```python
from build123d import *

# Parameters (mm, degrees)
F0_W     = 88.9
F0_H     = 57.15
F0_R     = 4.7625
F0_W_2   = 85.160196
F0_H_2   = 10.460668
F1_DEPTH = 3.175
F0_W_3   = 95.25
F0_H_3   = 63.5
F2_DEPTH = 19.05


with BuildPart() as f1:
    # F0 (on Top) → F1 (new body)
    with BuildSketch(Plane.XY):
        Rectangle(F0_W, F0_H)
        Polygon((-25.4, 3.175), (-25.4, 11.1125), (-17.4625, 11.1125), (-17.4625, 3.175), (-8.742713, 3.175), (-8.742713, -4.7625), (-17.4625, -4.7625), (-17.4625, -12.7), (-25.4, -12.7), (-25.4, -4.7625), (-33.3375, -4.7625), (-33.3375, 3.175), align=None, mode=Mode.SUBTRACT)
        with BuildLine():
            add(Edge.make_bspline(
                [(-0.483984, -3.476414), (-0.483984, -7.115989), (6.659766, -5.296201), (13.803516, -3.476414), (6.659766, -1.656627), (-0.483984, 0.163161), (-0.483984, -3.476414)],
                knots=[0, 0, 0, 2.094395, 2.094395, 4.18879, 4.18879, 6.283185, 6.283185, 6.283185], degree=2, weights=[1, 0.5, 1, 0.5, 1, 0.5, 1]))
        make_face(mode=Mode.SUBTRACT)
        with Locations((21.604328, -5.65704)):
            Circle(F0_R, mode=Mode.SUBTRACT)
        with Locations((36.5125, -11.1125)):
            Circle(F0_R, mode=Mode.SUBTRACT)
        with Locations((0, 20.904867)):
            Rectangle(F0_W_2, F0_H_2, mode=Mode.SUBTRACT)
    extrude(amount=-F1_DEPTH)

    # F0 (on Top) → F2 (join)
    with BuildSketch(Plane.XY):
        Rectangle(F0_W_3, F0_H_3)
        Rectangle(F0_W, F0_H, mode=Mode.SUBTRACT)
    extrude(amount=-F2_DEPTH)


solid = f1.part
```
The model under review builds one solid part; all positions refer to its coordinate system, in mm. A direction names the side the tool comes from. Give positions to 0.01 mm unless a question says otherwise; leave off trailing zeros. Write each loop counter-clockwise with the first axis right and the second up, starting at its lowest first coordinate (ties: lowest second). Pieces come first, ordered by that corner, then holes. Notation, with made-up numbers: (-14, 67.25) -> (-4, 67.25) arc R16 cw to (-4, 80.25) -> close; hole circle Ø7 at (45.25, 47). An arc over 180 degrees is marked (long way). Answer in a Markdown table with one row per item.
1) Clearance check with flat-ended pins moving along their axes: P1, Ø5, axis at x = 10.5, y = 5.5, coming from the +Z side; P2, Ø15, axis at x = 36.51, y = -11.11, coming from the -Z side (3 decimals). State where each tip first meets the part, or that it passes through.
Worked answers:
| item | result |
|---|---|
| P1 | z = 0 |
| P2 | z = -3.175 |
2) Add section B-B on y = 22. State the section outline as (x, z) points (3 decimals).
Worked answers:
| item | result |
|---|---|
| outline | (-47.625, -19.05) -> (-44.45, -19.05) -> (-44.45, -3.175) -> (-42.58, -3.175) -> (-42.58, 0) -> (-47.625, 0) -> close; (42.58, -3.175) -> (44.45, -3.175) -> (44.45, -19.05) -> (47.625, -19.05) -> (47.625, 0) -> (42.58, 0) -> close |
3) Add section D-D on x = -19.5. Count the separate pieces of the cut face and the enclosed holes in it, plus the area to 3 significant figures.
Worked answers:
| item | result |
|---|---|
| separate pieces | 3 |
| enclosed holes | 0 |
| area | 194 mm² |
4) For L1, parallel to X at y = 18.5, z = -3 (3 decimals); L2, parallel to X at y = 3, z = -4.25 (3 decimals); L3, parallel to Y at x = 0, z = -14.75 (3 decimals), list the stretches that pass through material, from the lowest coordinate up. Write a range as [from, to].
Worked answers:
| item | result |
|---|---|
| L1 | [-47.625, -42.58], [42.58, 47.625] |
| L2 | [-47.625, -44.45], [44.45, 47.625] |
| L3 | [-31.75, -28.575], [28.575, 31.75] |
5) Mouldability with a two-part tool opening along Y and no side actions: class faces 4 (the flat face through (-1, -31.75, -9)), 5 (the flat face through (-29, -4.762, -2)), 6 (the flat face through (-47.625, 0, -9)) as +Y half, -Y half, draft (parallel to the pull), parting line (faces both ways), or undercut.
Worked answers:
| item | result |
|---|---|
| face 4 | -Y half |
| face 5 | undercut |
| face 6 | draft |
6) Add section C-C on z = -6.25. State the section outline as (x, y) points (3 decimals).
Worked answers:
| item | result |
|---|---|
| outline | (-47.625, -31.75) -> (47.625, -31.75) -> (47.625, 31.75) -> (-47.625, 31.75) -> close; hole (-44.45, -28.575) -> (44.45, -28.575) -> (44.45, 28.575) -> (-44.45, 28.575) -> close |
7) Add section A-A on x = -2.5. State the section outline as (y, z) points (3 decimals), plus the area to 3 significant figures.
Worked answers:
| item | result |
|---|---|
| outline | (-31.75, -19.05) -> (-28.575, -19.05) -> (-28.575, -3.175) -> (15.675, -3.175) -> (15.675, 0) -> (-31.75, 0) -> close; (26.135, -3.175) -> (28.575, -3.175) -> (28.575, -19.05) -> (31.75, -19.05) -> (31.75, 0) -> (26.135, 0) -> close |
| area | 269 mm² |
8) Tool access review of faces 1 (the flat face through (-33.338, -1, -2)), 2 (the flat face through (-1, 0, 0)), 3 (the flat face through (-1, -28.575, -11)): name each direction out of +Z, -Z, +X, -X, +Y, -Y from which nothing blocks a thin tool from reaching the whole face with its end or side.
Worked answers:
| item | result |
|---|---|
| face 1 | +Z, -Z |
| face 2 | +Z, +X, -X, +Y, -Y |
| face 3 | -Z |
